Autodesk Inventor part; units mm, degrees
ref_plane "YZ Plane" through (0, 0, 0) normal (1, 0, 0) x (0, 1, 0)
ref_plane "XZ Plane" through (0, 0, 0) normal (0, 1, 0) x (-1, 0, 0)
ref_plane "XY Plane" through (0, 0, 0) normal (0, 0, 1) x (1, 0, 0)
sketch "Base" plane through (0, 0, 0) normal (0, 0, 1) x (1, 0, 0)
  line L0 (-152.6, 0) -> (152.6, 0) construction
  line L1 (0, -28.7) -> (0, 28.7) construction
  circle A0 centre (-95, 0) radius 3.5
  circle A1 centre (95, 0) radius 3.5
  line L2 (-109, 8.7447) -> (-109, 0)
  line L3 (-109, 8.7447) -> (-88, 14.3716)
  line L4 (-88, 14.3716) -> (-82.8577, 20.5)
  line L5 (-82.8577, 20.5) -> (0, 20.5)
  line L6 (-109, -8.7447) -> (-109, 0)
  line L7 (-109, -8.7447) -> (-88, -14.3716)
  line L8 (-88, -14.3716) -> (-82.8577, -20.5)
  line L9 (-82.8577, -20.5) -> (0, -20.5)
  line L10 (109, 8.7447) -> (109, 0)
  line L11 (109, 8.7447) -> (88, 14.3716)
  line L12 (88, 14.3716) -> (82.8577, 20.5)
  line L13 (82.8577, 20.5) -> (0, 20.5)
  line L14 (82.8577, -20.5) -> (0, -20.5)
  line L15 (88, -14.3716) -> (82.8577, -20.5)
  line L16 (109, -8.7447) -> (88, -14.3716)
  line L17 (109, -8.7447) -> (109, 0)
  circle A2 centre (-68, 9.5) radius 4
  line L18 (-58, 0) -> (-58, 20.5) construction
  line L19 (-68, 13.5) -> (-58, 13.5)
  circle A3 centre (-58, -7.8205) radius 4
  line L20 (-58, 0) -> (-58, -7.8205) construction
  line L21 (-71.4641, 7.5) -> (-61.4641, -9.8205)
  circle A4 centre (-48, 9.5) radius 4
  line L22 (-58, 13.5) -> (-48, 13.5)
  line L23 (-54.5359, -9.8205) -> (-44.5359, 7.5)
  circle A5 centre (-29, 9.5) radius 4
  circle A6 centre (-39, -7.8205) radius 4
  circle A7 centre (-19, -7.8205) radius 4
  line L24 (-48, 13.5) -> (-29, 13.5) construction
  line L25 (-39, -11.8205) -> (-19, -11.8205)
  line L26 (-42.4641, -5.8205) -> (-32.4641, 11.5)
  line L27 (-25.5359, 11.5) -> (-15.5359, -5.8205)
  line L28 (-58, -11.8205) -> (-39, -11.8205) construction
  line L29 (-29, 9.5) -> (-29, -11.8205) construction
  circle A8 centre (10, 9.5) radius 4
  line L30 (10, 13.5) -> (0, 13.5)
  circle A9 centre (0, -7.8205) radius 4
  line L31 (13.4641, 7.5) -> (3.4641, -9.8205)
  circle A10 centre (-10, 9.5) radius 4
  line L32 (0, 13.5) -> (-10, 13.5)
  line L33 (-3.4641, -9.8205) -> (-13.4641, 7.5)
  circle A11 centre (68, 9.5) radius 4
  line L34 (68, 13.5) -> (58, 13.5)
  circle A12 centre (58, -7.8205) radius 4
  line L35 (71.4641, 7.5) -> (61.4641, -9.8205)
  circle A13 centre (48, 9.5) radius 4
  line L36 (58, 13.5) -> (48, 13.5)
  line L37 (54.5359, -9.8205) -> (44.5359, 7.5)
  circle A14 centre (29, 9.5) radius 4
  circle A15 centre (39, -7.8205) radius 4
  circle A16 centre (19, -7.8205) radius 4
  line L38 (39, -11.8205) -> (19, -11.8205)
  line L39 (42.4641, -5.8205) -> (32.4641, 11.5)
  line L40 (25.5359, 11.5) -> (15.5359, -5.8205)
  point P0 (0, 0)
  point P1 (-58, 10.25)
  dimension "d0" = 7
  dimension "d1" = 190
  dimension "d3" = 130
  dimension "d4" = 165
  dimension "d5" = 8
  dimension "d7" = 218
  dimension "d8" = 41
  dimension "d12" = 21
  dimension "d14" = 8
  dimension "d15" = 8
  dimension "d16" = 20
  dimension "d17" = 60
  dimension "d18" = 7
  dimension "d20" = 8.4545
  dimension "d21" = 8.4545
extrude "BaseFeature" add sketch "Base" along normal blind 12
fillet "OutsideFilletsFeature" radius 4 12 edges at (-109, -8.7447, 6) (-109, 8.7447, 6) (-88, -14.3716, 6) (-82.8577, -20.5, 6) (-88, 14.3716, 6) (-82.8577, 20.5, 6) (82.8577, 20.5, 6) (88, 14.3716, 6) (109, -8.7447, 6) (88, -14.3716, 6) (82.8577, -20.5, 6) (109, 8.7447, 6)
properties part number "BatteryMount"
Verification items for the finished model (mm, model axes). A direction names the side the tool comes from. Coordinates: 2 decimals unless noted, no trailing zeros. Write each loop counter-clockwise with the first axis right and the second up, starting at its lowest first coordinate (ties: lowest second). Pieces come first, ordered by that corner, then holes. Notation, with made-up numbers: (9, 82) -> (53, 82) arc R22 ccw to (53, 112) -> close; hole circle Ø4 at (35, 76). An arc over 180 degrees is marked (long way). One line per item, written item: value. Start each with the question number.
Q1. Cross-section at B-B on y = 0. State how many separate pieces and enclosed holes the cut face has, and give its area (3 significant figures).
Q2. Cross-section at A-A on x = -93.5. Enter the section's corners in (y, z).
Q3. Mould release check, pull along X, two halves, no side actions. Record for faces 3 (the flat face through (-2, -13, 0)), 4 (the flat face through (-66.534, -1.039, 5.916)), 5 (the cylindrical face through (108.196, 8.081, 6.084)), 6 (the flat face through (0, 13.5, 6)): pulls with the +X half, pulls with the -X half, needs draft (parallel to the pull), parting line crosses it, or undercut.
Q4. Cross-section at D-D on x = -7.5. Enter the section's corners in (y, z).
Q5. Access from +Z, -Z, +X, -X, +Y, -Y to the whole of each face (thin tool, end or side, straight path). Record for faces 1 (the flat face through (85.645, 17.178, 5.916)), 2 (the cylindrical face through (-57.94, -11.82, 5.92)).
Q6. Thickness scan on L1, parallel to X at y = -5, z = 4.75; L2, parallel to Y at x = 29, z = 3.25; L3, parallel to Y at x = -95, z = 7.25. Record the ranges inside material, lowest first. Write a range as from..to.
Checked values:
1. separate pieces: 8
1. enclosed holes: 0
1. area: 1,310 mm²
2. outline: (-12.9, 0) -> (-3.16, 0) -> (-3.16, 12) -> (-12.9, 12) -> close; (3.16, 0) -> (12.9, 0) -> (12.9, 12) -> (3.16, 12) -> close
3. face 3: needs draft
3. face 4: undercut
3. face 5: pulls with the +X half
3. face 6: undercut
4. outline: (-20.5, 0) -> (-2.83, 0) -> (-2.83, 12) -> (-20.5, 12) -> close; (13.5, 0) -> (20.5, 0) -> (20.5, 12) -> (13.5, 12) -> close
5. face 1: +Z, -Z, +X, +Y
5. face 2: +Z, -Z
6. L1: x = -109..-64.25, -51.75..-41.99, -16.01..-6.25, 6.25..16.01, 41.99..51.75, 64.25..109
6. L2: y = -20.5..-11.82, 13.5..20.5
6. L3: y = -12.5..-3.5, 3.5..12.5
